Verification items for this drawing (mm, ordinates from the low corner). A direction names the side the tool comes from. Round coordinates to 2 decimals unless told otherwise and drop trailing zeros. Write each loop counter-clockwise with the first axis right and the second up, starting at its lowest first coordinate (ties: lowest second). Pieces come first, ordered by that corner, then holes. Notation, with made-up numbers: M -28.75,-33.5 L 22.25,-33.5 A29 ccw 22.25,-9.5 Z; hole C -21,16.5 d7. An arc over 180 degrees is marked long. Write each question's results on one line, items separated by ' | '.
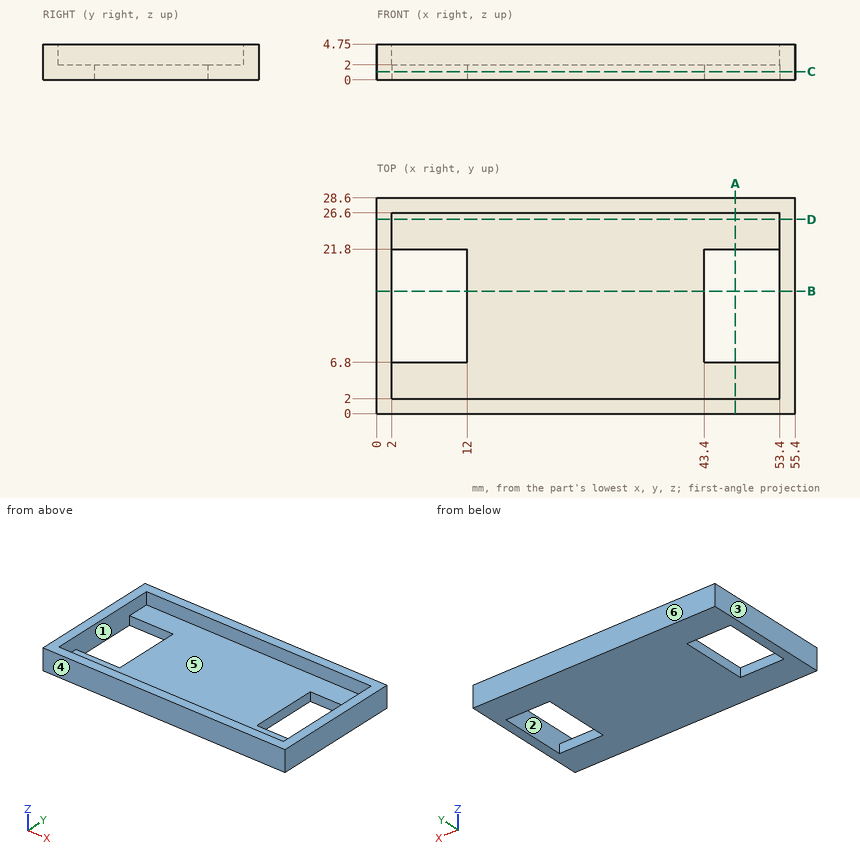
1) Depth check by flat-ended pin: P1, Ø12.5, axis at x = 21, y = 17, coming from the +Z side. Enter the tip coordinate at first touch or a pass-through.
Calculated:
P1: stops at z = 2
2) Draft check along X on the marked faces 1, 2, 3 and 4. Enter one of: pulls with the +X half, pulls with the -X half, needs draft (parallel to the pull), parting line crosses it, or undercut.
Calculated:
face 1: undercut | face 2: undercut | face 3: pulls with the -X half | face 4: needs draft
3) Access from +Z, -Z, +X, -X, +Y, -Y to the whole of each face (thin tool, end or side, straight path). Record for the marked faces 5 and 6.
Calculated:
face 5: +Z | face 6: +Z, -Z, +X, -X, +Y
4) Material ranges on line 1 (X direction, y = 14.75, z = 0.6); line 2 (Y direction, x = 28, z = 3.1); line 3 (X direction, y = 16.5, z = 2.35), recorded low to high. Write a range as [from, to].
Calculated:
line 1: x = [0, 2], [12, 43.4], [53.4, 55.4] | line 2: y = [0, 2], [26.6, 28.6] | line 3: x = [0, 2], [53.4, 55.4]
5) Sectioned sample at D-D, the plane y = 25.75. Record the cut outline in (x, z), and give its area (3 significant figures).
Calculated:
outline: M 0,0 L 55.4,0 L 55.4,4.75 L 53.4,4.75 L 53.4,2 L 2,2 L 2,4.75 L 0,4.75 Z | area: 122 mm²
6) Sectioned sample at A-A, the plane x = 47.5. Record the cut outline in (y, z), and give its area (3 significant figures).
Calculated:
outline: M 0,0 L 6.8,0 L 6.8,2 L 2,2 L 2,4.75 L 0,4.75 Z; M 21.8,0 L 28.6,0 L 28.6,4.75 L 26.6,4.75 L 26.6,2 L 21.8,2 Z | area: 38.2 mm²
7) Sectioned sample at B-B, the plane y = 16.25. Record the cut outline in (x, z).
Calculated:
outline: M 0,0 L 2,0 L 2,4.75 L 0,4.75 Z; M 12,0 L 43.4,0 L 43.4,2 L 12,2 Z; M 53.4,0 L 55.4,0 L 55.4,4.75 L 53.4,4.75 Z
8) Sectioned sample at C-C, the plane z = 1.1. Record the cut outline in (x, y).
Calculated:
outline: M 0,0 L 55.4,0 L 55.4,28.6 L 0,28.6 Z; hole M 2,6.8 L 12,6.8 L 12,21.8 L 2,21.8 Z; hole M 43.4,6.8 L 53.4,6.8 L 53.4,21.8 L 43.4,21.8 Z
